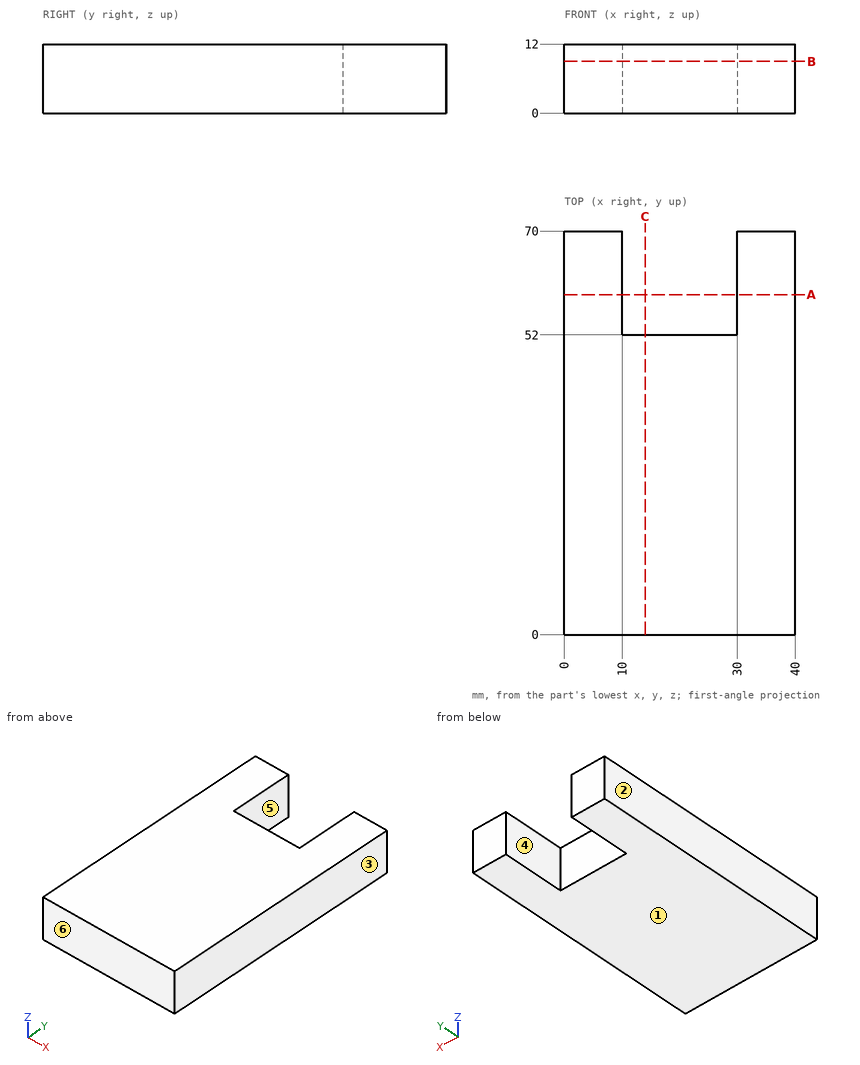
Answer from the drawing. Dimensions are ordinates in mm from the lowest x, y and z of the part. A direction names the side the tool comes from. Give positions to 0.01 mm unless a question says otherwise; leave off trailing zeros. Order: outer loops, then holes, each group sorted by start corner. A loop starts at its lowest first (then second) coordinate and runs counter-clockwise, first axis right, second up. Notation, with made-up numbers: (-25.5, 81.25) -> (-19.5, 81.25) arc R17 ccw to (-19.5, 97.25) -> close; hole circle Ø1 at (-18, -25.5). An arc over 180 degrees is marked (long way). One line per item, written item: value.
Item 1: Determine the mould class of the marked faces 1, 2, 3 and 4 for opening direction X: released by +X, released by -X, zero draft, split by the parting line, or undercut.
Answer sheet:
face 1: zero draft
face 2: released by -X
face 3: released by +X
face 4: undercut
Item 2: Find section C-C, the plane x = 14. Give the vertices of the cut face in (y, z).
Answer sheet:
outline: (0, 0) -> (52, 0) -> (52, 12) -> (0, 12) -> close
Item 3: Straight lines are drawn through the part: probe 1 along X at (y, z) = (66.5, 4.25); probe 2 along Y at (x, z) = (24, 2.5). For each, find the intervals that lie inside material, in ascending order.
Answer sheet:
probe 1: 0 to 10, 30 to 40
probe 2: 0 to 52
Item 4: Find section B-B, the plane z = 9. Give the vertices of the cut face in (x, y), plus the area to 3 significant figures.
Answer sheet:
outline: (0, 0) -> (40, 0) -> (40, 70) -> (30, 70) -> (30, 52) -> (10, 52) -> (10, 70) -> (0, 70) -> close
area: 2,440 mm²
Item 5: A flat-ended cylindrical pin translates along its axis: P1, Ø6, axis at x = 15.5, z = 5.5, coming from the +Y side. Find the tip coordinate at first contact, or state that the pin passes through.
Answer sheet:
P1: y = 52
Item 6: Find section A-A, the plane y = 59. Give the vertices of the cut face in (x, z).
Answer sheet:
outline: (0, 0) -> (10, 0) -> (10, 12) -> (0, 12) -> close; (30, 0) -> (40, 0) -> (40, 12) -> (30, 12) -> close
Item 7: A tool of negligible diameter and unlimited length cuts with its end or side. For the marked faces 5 and 6, from which of +Z, -Z, +X, -X, +Y, -Y can it reach the whole face along a straight path? Write none if from no direction.
Answer sheet:
face 5: +Z, -Z, +Y
face 6: +Z, -Z, +X, -X, -Y
